from build123d import *

# Parameters (mm, degrees)
SKETCH1_R           = 22.225
BOSS_EXTRUDE1_DEPTH = 101.6
FILLET1_R           = 2.54
SKETCH2_R           = 2.1828125
CUT_EXTRUDE1_DEPTH  = 6.858


with BuildPart() as part:
    # Sketch1 → Boss-Extrude1 (new body)
    with BuildSketch(Plane(origin=(0, 0, 0), x_dir=(1, 0, 0), z_dir=(0, 1, 0))):
        Circle(SKETCH1_R)
    extrude(amount=BOSS_EXTRUDE1_DEPTH)

    # Fillet1
    fillet1_edges = [part.edges().sort_by_distance(p)[0] for p in [
        (-22.225, 101.6, 0),
    ]]
    fillet(fillet1_edges, radius=FILLET1_R)

    # Sketch2 → Cut-Extrude1 (cut)
    with BuildSketch(Plane(origin=(0, 101.6, 0), x_dir=(1, 0, 0), z_dir=(0, 1, 0))):
        Circle(SKETCH2_R)
    extrude(amount=-CUT_EXTRUDE1_DEPTH, mode=Mode.SUBTRACT)


solid = part.part
Geometry check sheet. Reference: the model listing, model coordinates, mm. A direction names the side the tool comes from. Round coordinates to 2 decimals unless told otherwise and drop trailing zeros. Write each loop counter-clockwise with the first axis right and the second up, starting at its lowest first coordinate (ties: lowest second). Pieces come first, ordered by that corner, then holes. Notation, with made-up numbers: (50, 84) -> (107, 84) arc R29 ccw to (107, 123) -> close; hole circle Ø1 at (12, -9.5). An arc over 180 degrees is marked (long way). One line per item, written item: value. Start each with the question number.
(1) Cross-section at A-A, the plane y = 9.5. Record the cut outline in (x, z) (3 decimals).
(2) Go/stop test with flat-tipped pins: pin 1 Ø1 at (y, z) = (30, 5) entering from +X; pin 2 Ø1.3 at (x, z) = (-1, 0) entering from +Y; pin 3 Ø5 at (x, y) = (12.5, 27.5) entering from +Z. Record where each tip stops, or that it passes through.
(3) Draft check along X on faces 1 (the cylindrical face through (-1.73, 98.22, 1.33)), 2 (the cylindrical face through (21.199, 48.837, -6.676)), 3 (the flat face through (0, 101.6, 4)). Enter one of: +X half, -X half, draft (parallel to the pull), parting line (faces both ways), or undercut.
(4) Scan lines: line 1 (X direction, y = 96, z = 0) (3 decimals); line 2 (X direction, y = 99.75, z = 0); line 3 (Z direction, x = 9.5, y = 35.5). Record each from-to range of solid material in increasing order. Write a range as [from, to].
(5) Access from +Z, -Z, +X, -X, +Y, -Y to the whole of each face (thin tool, end or side, straight path). Record for faces 4 (the flat face through (0, 0, 0)), 5 (the flat face through (0, 94.742, 0)).
Answer:
1. outline: circle Ø44.45 at (0, 0)
2. pin 1: x = 21.76
2. pin 2: y = 94.74
2. pin 3: z = 19.85
3. face 1: undercut
3. face 2: parting line
3. face 3: draft
4. line 1: [-22.225, -2.183], [2.183, 22.225]
4. line 2: [-22.13, -2.18], [2.18, 22.13]
4. line 3: [-20.09, 20.09]
5. face 4: +Z, -Z, +X, -X, -Y
5. face 5: +Y
